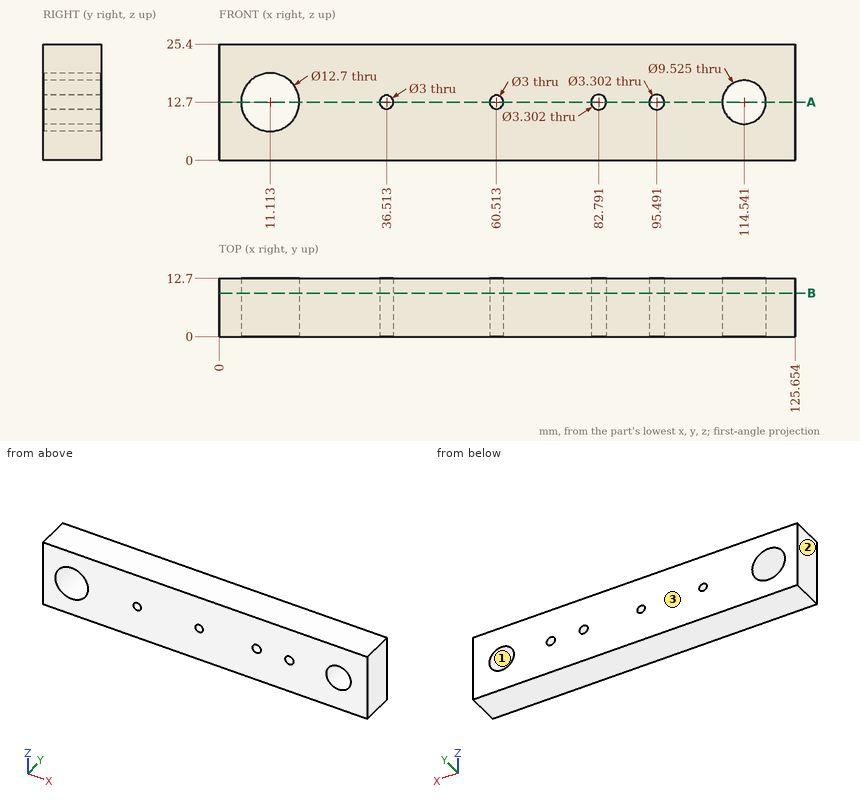
Answer from the drawing. Dimensions are ordinates in mm from the lowest x, y and z of the part. Give positions to 0.01 mm unless a question says otherwise; leave off trailing zeros. Loops run counter-clockwise (first coordinate to the right, second up) from the corner with the lowest first, then second, coordinate; pieces in that order, holes last. Notation, with made-up numbers: (-5.5, 16) - (11.5, 16) arc R21 ccw to (11.5, 52) - close; hole circle Ø4 at (12.25, 52). An arc over 180 degrees is marked (long way). Answer as a JSON object with one key per item and string values.
1. Find the intervals of material crossed by L1, parallel to Z at x = 111, y = 9.75 (1 decimal); L2, parallel to X at y = 10.75, z = 16.5 (1 decimal); L3, parallel to Z at x = 116, y = 3 (1 decimal), in increasing order. Write a range as [from, to].
Determined:
{"L1": "[0, 9.5], [15.9, 25.4]", "L2": "[0, 6], [16.2, 111.7], [117.4, 125.7]", "L3": "[0, 8.2], [17.2, 25.4]"}
2. A cutting plane is placed at B-B (y = 9.5). Give the number of separate pieces and of enclosed holes in the cut face, then the cut area to 3 significant figures.
Determined:
{"separate pieces": "1", "enclosed holes": "6", "area": "2,960 mm²"}
3. A flat-ended cylindrical pin translates along its axis: pin 1 Ø5 at (x, z) = (36.51, 12.7) entering from +Y. Find the tip coordinate at first contact, or state that the pin passes through.
Determined:
{"pin 1": "y = 12.7"}
4. A cutting plane is placed at A-A (z = 12.7). Write down the section's boundary in (x, y).
Determined:
{"outline": "(0, 0) - (4.76, 0) - (4.76, 12.7) - (0, 12.7) - close; (17.46, 0) - (35.01, 0) - (35.01, 12.7) - (17.46, 12.7) - close; (38.01, 0) - (59.01, 0) - (59.01, 12.7) - (38.01, 12.7) - close; (62.01, 0) - (81.14, 0) - (81.14, 12.7) - (62.01, 12.7) - close; (84.44, 0) - (93.84, 0) - (93.84, 12.7) - (84.44, 12.7) - close; (97.14, 0) - (109.78, 0) - (109.78, 12.7) - (97.14, 12.7) - close; (119.3, 0) - (125.65, 0) - (125.65, 12.7) - (119.3, 12.7) - close"}
5. For a pull along X with two mould halves and no side action, classify the marked faces 1, 2 and 3 as pulls with the +X half, pulls with the -X half, needs draft (parallel to the pull), parting line crosses it, or undercut.
Determined:
{"face 1": "undercut", "face 2": "pulls with the -X half", "face 3": "needs draft"}
